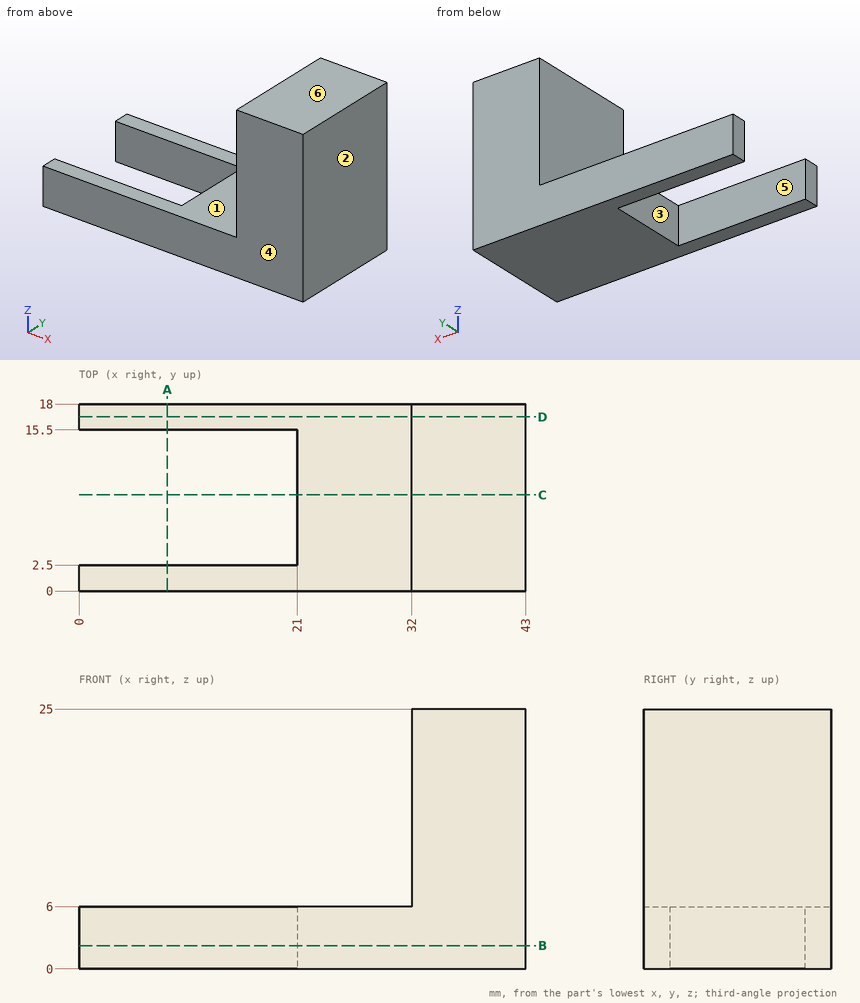
Study the drawing (mm; zero at the part's minimum x, y, z) and answer. A direction names the side the tool comes from. Coordinates: 2 decimals unless noted, no trailing zeros. Write each loop counter-clockwise with the first axis right and the second up, starting at its lowest first coordinate (ties: lowest second). Pieces come first, ordered by that corner, then holes. Notation, with made-up numbers: (77, -33) -> (135, -33) arc R14 ccw to (135, -28) -> close; hole circle Ø11 at (-14.75, 7). An arc over 180 degrees is marked (long way). Write each question's results on one line, items separated by ' | '. Start each with the question number.
1) A cutting plane is placed at A-A (x = 8.5). Determine the outline of the cut face in (y, z).
2) Flat-ended cylindrical pins translate along their axes: pin 1 Ø4 at (y, z) = (8.5, 13.5) entering from -X; pin 2 Ø1.8 at (y, z) = (9, 2) entering from -X; pin 3 Ø6 at (x, y) = (26, 16) entering from +Z. Find the tip coordinate at first contact, or state that the pin passes through.
3) Straight lines are drawn through the part: probe 1 along Y at (x, z) = (17, 3); probe 2 along Z at (x, y) = (30, 14.75); probe 3 along X at (y, z) = (16.75, 21). For each, find the intervals that lie inside material, in ascending order.
4) A cutting plane is placed at D-D (y = 16.75). Determine the outline of the cut face in (x, z).
5) A cutting plane is placed at B-B (z = 2.25). Determine the outline of the cut face in (x, y), then the cut area to 3 significant figures.
6) A tool of negligible diameter and unlimited length cuts with its end or side. For the marked faces 1, 2 and 3, from which of +Z, -Z, +X, -X, +Y, -Y can it reach the whole face along a straight path? Write none if from no direction.
7) For a pull along Y with two mould halves and no side action, classify the marked faces 4, 5 and 6 as +Y half, -Y half, draft (parallel to the pull), parting line (faces both ways), or undercut.
8) A cutting plane is placed at C-C (y = 9.25). Determine the outline of the cut face in (x, z), then the cut area to 3 significant figures.
Values follow:
1) outline: (0, 0) -> (2.5, 0) -> (2.5, 6) -> (0, 6) -> close; (15.5, 0) -> (18, 0) -> (18, 6) -> (15.5, 6) -> close
2) pin 1: x = 32 | pin 2: x = 21 | pin 3: z = 6
3) probe 1: 0 to 2.5, 15.5 to 18 | probe 2: 0 to 6 | probe 3: 32 to 43
4) outline: (0, 0) -> (43, 0) -> (43, 25) -> (32, 25) -> (32, 6) -> (0, 6) -> close
5) outline: (0, 0) -> (43, 0) -> (43, 18) -> (0, 18) -> (0, 15.5) -> (21, 15.5) -> (21, 2.5) -> (0, 2.5) -> close | area: 501 mm²
6) face 1: +Z, -X, +Y, -Y | face 2: +Z, -Z, +X, +Y, -Y | face 3: +Z, -Z, -X
7) face 4: -Y half | face 5: undercut | face 6: draft
8) outline: (21, 0) -> (43, 0) -> (43, 25) -> (32, 25) -> (32, 6) -> (21, 6) -> close | area: 341 mm²
